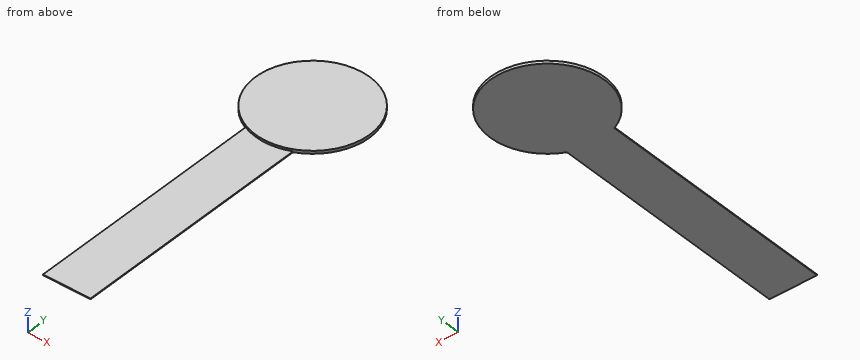
```python
from build123d import *

# Parameters (mm, degrees)
SKETCH1_R           = 9.15
BOSS_EXTRUDE1_DEPTH = 0.46
SKETCH2_W           = 7.62
SKETCH2_H           = 38.870961594
BOSS_EXTRUDE2_DEPTH = 0.13


with BuildPart() as part:
    # Sketch1 → Boss-Extrude1 (new body)
    with BuildSketch(Plane.XY):
        Circle(SKETCH1_R)
    extrude(amount=BOSS_EXTRUDE1_DEPTH)

    # Sketch2 → Boss-Extrude2 (add)
    with BuildSketch(Plane.XY):
        with Locations((0, -27.754519203)):
            Rectangle(SKETCH2_W, SKETCH2_H)
    extrude(amount=BOSS_EXTRUDE2_DEPTH)


solid = part.part
```
Model file for the job. Use its own axes, mm. Give positions to 0.01 mm unless a question says otherwise; leave off trailing zeros. Loops run counter-clockwise (first coordinate to the right, second up) from the corner with the lowest first, then second, coordinate; pieces in that order, holes last. Notation, with made-up numbers: (18.5, 7) - (23.5, 7) arc R10 ccw to (23.5, 20) - close; hole circle Ø10 at (4, -3.75). An arc over 180 degrees is marked (long way). One line per item, written item: value. Start each with the question number.
1. Slice it at D-D (y = -3). List the corners of the cut face in (x, z), plus the area to 3 significant figures.
2. Slice it at B-B (y = -20). List the corners of the cut face in (x, z).
3. Probe L1, parallel to Y at x = 0.25, z = 0.4; L2, parallel to Y at x = 8, z = 0.4; L3, parallel to X at y = 6.5, z = 0.15. List the from-to ranges inside material, lowest first. Write a range as from..to.
4. Slice it at A-A (x = 0). List the corners of the cut face in (y, z).
5. Pin check, flat tip, straight feed: pin 1 (6 mm diameter, centred on x = -1, y = -35, fed in from +Z). Stop position of the tip, or through.
6. Slice it at C-C (z = 0.25). List the corners of the cut face in (x, y), plus the area to 3 significant figures.
Solution:
1. outline: (-8.64, 0) - (8.64, 0) - (8.64, 0.46) - (-8.64, 0.46) - close
1. area: 7.95 mm^2
2. outline: (-3.81, 0) - (3.81, 0) - (3.81, 0.13) - (-3.81, 0.13) - close
3. L1: y = -9.15..9.15
3. L2: y = -4.44..4.44
3. L3: x = -6.44..6.44
4. outline: (-47.19, 0) - (9.15, 0) - (9.15, 0.46) - (-9.15, 0.46) - (-9.15, 0.13) - (-47.19, 0.13) - close
5. pin 1: stops at z = 0.13
6. outline: circle Ø18.3 at (0, 0)
6. area: 263 mm^2
